```python
from build123d import *

# Parameters (mm, degrees)
MAIN_DEPTH      = 10
FILLET1_R       = 2
FILLET2_R       = 2
SKETCH2_R       = 1.25
BOLT_SLOT_DEPTH = 3
SKETCH3_W       = 5
SKETCH3_H       = 13
FRONT_TAB_DEPTH = 2
SKETCH4_W       = 1.5
SKETCH4_H       = 5
TOP_TAB_DEPTH   = 2
FILLET3_R       = 2
FILLET4_R       = 2


with BuildPart() as part:
    # Sketch1 → main (new body)
    with BuildSketch(Plane(origin=(0, 0, 0), x_dir=(0, 0, -1), z_dir=(1, 0, 0))):
        Polygon((-9, 0), (9, 0), (9, -10), (16, -10), (16, -13), (6, -13), (6, -3), (-6, -3), (-6, -13), (-16, -13), (-16, -10), (-9, -10), align=None)
    extrude(amount=MAIN_DEPTH)

    # Fillet1
    fillet1_edges = [part.edges().sort_by_distance(p)[0] for p in [
        (5, -13, 6),
    ]]
    fillet(fillet1_edges, radius=FILLET1_R)

    # Fillet2
    fillet2_edges = [part.edges().sort_by_distance(p)[0] for p in [
        (5, -13, -6),
    ]]
    fillet(fillet2_edges, radius=FILLET2_R)

    # Sketch2 → bolt slot (cut)
    with BuildSketch(Plane.XZ.offset(13)):
        with Locations(Location((5, 12, 0), (0, 0, 270))):
            Circle(SKETCH2_R)
        with Locations(Location((5, -12, 0), (0, 0, 270))):
            Circle(SKETCH2_R)
    extrude(amount=-BOLT_SLOT_DEPTH, mode=Mode.SUBTRACT)

    # Sketch3 → front tab (add)
    with BuildSketch(Plane.ZY):
        with Locations((-6.5, -6.5)):
            Rectangle(SKETCH3_W, SKETCH3_H)
        with Locations((6.5, -6.5)):
            Rectangle(SKETCH3_W, SKETCH3_H)
    extrude(amount=FRONT_TAB_DEPTH)

    # Sketch4 → top tab (add)
    with BuildSketch(Plane.XZ.offset(3)):
        with Locations((7.25, -3.5)):
            Rectangle(SKETCH4_W, SKETCH4_H)
    extrude(amount=TOP_TAB_DEPTH)

    # Fillet3
    fillet3_edges = [part.edges().sort_by_distance(p)[0] for p in [
        (4, 0, -9),
    ]]
    fillet(fillet3_edges, radius=FILLET3_R)

    # Fillet4
    fillet4_edges = [part.edges().sort_by_distance(p)[0] for p in [
        (4, 0, 9),
    ]]
    fillet(fillet4_edges, radius=FILLET4_R)


solid = part.part
```
Here's how the part is built. I have some questions about the finished solid (model axes, mm). A direction names the side the tool comes from. Round coordinates to 2 decimals unless told otherwise and drop trailing zeros. Order: outer loops, then holes, each group sorted by start corner. A loop starts at its lowest first (then second) coordinate and runs counter-clockwise, first axis right, second up. Notation, with made-up numbers: (2, 4) -> (51, 4) arc R15 cw to (51, 22) -> close; hole circle Ø2 at (-32.75, 53). An arc over 180 degrees is marked (long way). Use a Markdown table: item, result. Add a question column.
(1) If we mould it in two halves opening along Z, with no side actions, what happens to faces 1 (the face through (4, 0, 0)), 2 (the face through (0, -8, -5)), 3 (the face through (4.08, -0.57, 8.4))? For each: released by +Z, released by -Z, zero draft, split by the parting line, or undercut.
(2) Suppose I cut it at D-D, the plane x = 3.25. Please give me the cut outline in (y, z), and give its area (3 significant figures).
(3) Suppose I cut it at C-C, the plane y = -5.75. Please give me the cut outline in (x, z), and give its area (3 significant figures).
(4) For faces 4 (the face through (0, -8, 5)), 5 (the face through (7, -4, -1)), 6 (the face through (0, -11, -13)), 7 (the face through (-1, -7, 4)), 8 (the face through (4, -10, 13)), which set-ups out of +Z, -Z, +X, -X, +Y, -Y let a thin tool reach every point of the face, with its end or its side?
(5) For pin 1 Ø4 at (x, z) = (6, -12) entering from +Y; pin 2 Ø3 at (x, y) = (5.5, -7) entering from +Z; pin 3 Ø1.5 at (y, z) = (-8.5, -4.5) entering from +X, each with a flat end and sliding along its axis, tell me the tip position at first contact or that it passes through.
(6) Suppose I cut it at B-B, the plane z = -12. Please give me the cut outline in (x, y), and give its area (3 significant figures).
(7) I need wall thicknesses on line 1 along X through (y, z) = (-10.55, -12); line 2 along Z through (x, y) = (4.75, -11.5); line 3 along Z through (x, y) = (4.5, -11.75). Which ranges of each line are inside material? Lowest first, please.
(8) Suppose I cut it at A-A, the plane x = 5. Please give me the cut outline in (y, z), and give its area (3 significant figures).
Verdict:
| question | item | result |
|---|---|---|
| 1 | face 1 | zero draft |
| 1 | face 2 | undercut |
| 1 | face 3 | released by +Z |
| 2 | outline | (-13, -16) -> (-10, -16) -> (-10, -9) -> (-2, -9) arc R2 ccw to (0, -7) -> (0, 7) arc R2 ccw to (-2, 9) -> (-10, 9) -> (-10, 16) -> (-13, 16) -> (-13, 8) arc R2 ccw to (-11, 6) -> (-3, 6) -> (-3, -6) -> (-11, -6) arc R2 ccw to (-13, -8) -> close |
| 2 | area | 153 mm2 |
| 3 | outline | (-2, -9) -> (10, -9) -> (10, -6) -> (0, -6) -> (0, -4) -> (-2, -4) -> close; (-2, 4) -> (0, 4) -> (0, 6) -> (10, 6) -> (10, 9) -> (-2, 9) -> close |
| 3 | area | 80.0 mm2 |
| 4 | face 4 | +X, -Y |
| 4 | face 5 | +X, -X, -Y |
| 4 | face 6 | -Z, -X, +Y, -Y |
| 4 | face 7 | -X, +Y, -Y |
| 4 | face 8 | +Z, +X, -X, +Y |
| 5 | pin 1 | y = -10 |
| 5 | pin 2 | z = 9 |
| 5 | pin 3 | x = 0 |
| 6 | outline | (0, -13) -> (3.75, -13) -> (3.75, -10) -> (0, -10) -> close; (6.25, -13) -> (10, -13) -> (10, -10) -> (6.25, -10) -> close |
| 6 | area | 22.5 mm2 |
| 7 | line 1 | 0 to 3.75, 6.25 to 10 |
| 7 | line 2 | -16 to -13.22, -10.78 to -6.06, 6.06 to 10.78, 13.22 to 16 |
| 7 | line 3 | -16 to -13.15, -10.85 to -6.15, 6.15 to 10.85, 13.15 to 16 |
| 8 | outline | (-13, -16) -> (-10, -16) -> (-10, -13.25) -> (-13, -13.25) -> close; (-13, -10.75) -> (-10, -10.75) -> (-10, -9) -> (-2, -9) arc R2 ccw to (0, -7) -> (0, 7) arc R2 ccw to (-2, 9) -> (-10, 9) -> (-10, 10.75) -> (-13, 10.75) -> (-13, 8) arc R2 ccw to (-11, 6) -> (-3, 6) -> (-3, -6) -> (-11, -6) arc R2 ccw to (-13, -8) -> close; (-13, 13.25) -> (-10, 13.25) -> (-10, 16) -> (-13, 16) -> close |
| 8 | area | 138 mm2 |
